Check sheet for the modelled part. Datum: model origin and axes. Units: mm. A direction names the side the tool comes from. Give positions to 0.01 mm unless a question says otherwise; leave off trailing zeros. Order: outer loops, then holes, each group sorted by start corner. A loop starts at its lowest first (then second) coordinate and runs counter-clockwise, first axis right, second up. Notation, with made-up numbers: M 71,14 L 87,14 A34 cw 87,47 Z; hole C 33.5,37.5 d4. An arc over 180 degrees is marked long. One line per question, with ' | ' between items. Start each with the question number.
Autodesk Inventor part; units mm, degrees
ref_plane "YZ Plane" through (0, 0, 0) normal (1, 0, 0) x (0, 1, 0)
ref_plane "XZ Plane" through (0, 0, 0) normal (0, 1, 0) x (-1, 0, 0)
ref_plane "XY Plane" through (0, 0, 0) normal (0, 0, 1) x (1, 0, 0)
sketch "Sketch1" plane through (0, 0, 0) normal (0, 1, 0) x (-1, 0, 0)
  line L0 (2.5675, -34.392) -> (-2.0625, -34.392)
  line L1 (-4.0625, -32.392) -> (-4.0625, 32.768)
  line L2 (-2.0625, 34.768) -> (2.5675, 34.768)
  line L3 (4.5675, 32.768) -> (4.5675, -32.392)
  arc A0 (4.5675, 32.768) -> (2.5675, 34.768) centre (2.5675, 32.768) ccw
  arc A1 (-2.0625, 34.768) -> (-4.0625, 32.768) centre (-2.0625, 32.768) ccw
  arc A2 (-4.0625, -32.392) -> (-2.0625, -34.392) centre (-2.0625, -32.392) ccw
  arc A3 (2.5675, -34.392) -> (4.5675, -32.392) centre (2.5675, -32.392) ccw
  point P0 (0, 0)
  point P1 (-4.0625, 34.768)
  point P2 (-4.0625, -34.392)
  point P3 (4.5675, 34.768)
  dimension "d0" = 8.63
  dimension "d1" = 69.16
  dimension "d2" = 2
extrude "Extrusion1" add sketch "Sketch1" along normal blind 6.35
sketch "Sketch2" plane through (0, 6.35, 0) normal (0, 1, 0) x (1, 0, 0)
  circle A0 centre (0, -31.355) radius 1.625
  circle A1 centre (0, 31.355) radius 1.625
  point P0 (0, 0)
  dimension "d5" = 3.25
  dimension "d6" = 3.25
  dimension "d7" = 31.355
  dimension "d8" = 31.355
extrude "Extrusion2" cut sketch "Sketch2" against normal blind 6.35
sketch "Sketch3" plane through (0, 6.35, 0) normal (0, 1, 0) x (1, 0, 0)
  line L0 (-2.569, -27.838) -> (2.061, -27.838)
  line L1 (4.061, -25.838) -> (4.061, 25.462)
  line L2 (2.061, 27.462) -> (-2.569, 27.462)
  line L3 (-4.569, 25.462) -> (-4.569, -25.838)
  line L4 (-2.5675, -34.768) -> (2.0625, -34.768)
  arc A0 (-4.569, -25.838) -> (-2.569, -27.838) centre (-2.569, -25.838) ccw
  arc A1 (2.061, -27.838) -> (4.061, -25.838) centre (2.061, -25.838) ccw
  arc A2 (4.061, 25.462) -> (2.061, 27.462) centre (2.061, 25.462) ccw
  arc A3 (-2.569, 27.462) -> (-4.569, 25.462) centre (-2.569, 25.462) ccw
  point P0 (0, 0)
  point P1 (4.061, 27.462)
  point P2 (4.061, -27.838)
  point P3 (-4.569, 27.462)
  dimension "d11" = 8.63
  dimension "d12" = 55.3
  dimension "d13" = 6.93
  dimension "d14" = 2
extrude "Extrusion3" add sketch "Sketch3" along normal blind 5.28
sketch "Sketch4" plane through (0, 11.63, 0) normal (0, 1, 0) x (1, 0, 0)
  line L0 (2.5, 25.855) -> (-2.5, 25.855)
  line L1 (-2.5, 25.855) -> (-2.5, -25.855)
  line L2 (-2.5, -25.855) -> (2.5, -25.855)
  line L3 (2.5, -25.855) -> (2.5, 25.855)
  line L4 (2.5, 25.855) -> (-2.5, -25.855) construction
  line L5 (-2.5, 25.855) -> (2.5, -25.855) construction
  point P0 (0, 0)
  dimension "d17" = 5
  dimension "d18" = 51.71
extrude "Extrusion4" cut sketch "Sketch4" against normal blind 11.63
chamfer "Chamfer1" distance 1 angle 45 4 edges at (-2.5, 11.63, 0) (0, 11.63, 25.855) (2.5, 11.63, 0) (0, 11.63, -25.855)
sketch "Sketch5" plane through (0, 0, 0) normal (0, -1, 0) x (1, 0, 0)
  point P0 (0, 0)
Item 1: Section check C-C, the plane y = 3. State how many separate pieces and enclosed holes the cut face has, then the cut area to 3 significant figures.
Item 2: Go/stop test with flat-tipped pins: P1, Ø1.5, axis at x = 2, z = -10, coming from the -Y side; P2, Ø3, axis at x = 3, y = 8.5, coming from the -Z side; P3, Ø5, axis at x = 0, z = -31.355, coming from the +Y side; P4, Ø2.5, axis at x = -1, y = 10, coming from the +Z side. Record where each tip stops, or that it passes through.
Item 3: Set-up check for faces 1 (the face through (-4, 8.95, -26.86)), 2 (the face through (0, 9, 27.838)), 3 (the face through (0, 9, -27.462)), 4 (the face through (2.5, 5, 0)): record each of +Z, -Z, +X, -X, +Y, -Y from which the full face is reachable in a straight line by a thin tool's end or side.
Item 4: Draft check along Z on faces 5 (the face through (0, 5, -25.855)), 6 (the face through (-3.968, 8.953, 27.268)), 7 (the face through (0, 3, -34.392)). Enter one of: released by +Z, released by -Z, zero draft, split by the parting line, or undercut.
Item 5: Section check A-A, the plane x = 0. Record the cut outline in (y, z) (3 decimals), then the cut area to 3 significant figures.
Item 6: Scan lines: probe 1 along Z at (x, y) = (0, 1.5) (3 decimals); probe 2 along X at (y, z) = (2, -18.5); probe 3 along Z at (x, y) = (2, 3) (3 decimals). Record each from-to range of solid material in increasing order. Write a range as [from, to].
Reported:
1) separate pieces: 1 | enclosed holes: 3 | area: 318 mm^2
2) P1: stops at y = 0 | P2: stops at z = -27.46 | P3: stops at y = 6.35 | P4: stops at z = 27.84
3) face 1: -Z, -X, +Y | face 2: +Z, +X, -X, +Y | face 3: -Z, +X, -X, +Y | face 4: +Y, -Y
4) face 5: undercut | face 6: released by +Z | face 7: released by -Z
5) outline: M 0,-34.392 L 6.35,-34.392 L 6.35,-32.98 L 0,-32.98 Z; M 0,-29.73 L 6.35,-29.73 L 6.35,-27.462 L 11.63,-27.462 L 11.63,-26.852 L 10.633,-25.855 L 0,-25.855 Z; M 0,25.855 L 10.633,25.855 L 11.63,26.852 L 11.63,27.838 L 6.35,27.838 L 6.35,29.73 L 0,29.73 Z; M 0,32.98 L 6.35,32.98 L 6.35,34.768 L 0,34.768 Z | area: 87.5 mm^2
6) probe 1: z = [-34.392, -32.98], [-29.73, -25.855], [25.855, 29.73], [32.98, 34.768] | probe 2: x = [-4.57, -2.5], [2.5, 4.06] | probe 3: z = [-34.392, -25.855], [25.855, 34.768]
